```python
from build123d import *

# Parameters (mm, degrees)
F0_W     = 114.3
F0_H     = 152.4
F1_DEPTH = 15.24
F2_W     = 101.6
F2_H     = 14.1132464528
F3_DEPTH = 57.15
F4_DEPTH = 57.15
F6_DEPTH = 50.8
F7_DEPTH = 100.838


with BuildPart() as f1:
    # F0 (on Right) → F1 (new body)
    with BuildSketch(Plane.YZ):
        Rectangle(F0_W, F0_H)
    extrude(amount=F1_DEPTH)

    # F2 (on Front) → F3 (join)
    with BuildSketch(Plane.XZ):
        with Locations((66.04, -69.1433767736)):
            Rectangle(F2_W, F2_H)
    extrude(amount=F3_DEPTH)

    # F2 (on Front) → F4 (join)
    with BuildSketch(Plane.XZ):
        with Locations((66.04, -69.1433767736)):
            Rectangle(F2_W, F2_H)
    extrude(amount=-F4_DEPTH)

    # F5 (on Front) → F6 (join)
    with BuildSketch(Plane.XZ):
        with BuildLine():
            ThreePointArc((100.9056121111, 15.8293191344), (108.7441404523, 44.1781850532), (100.9056121111, 72.527050972))
            ThreePointArc((100.9056121111, 72.527050972), (58.597203119, 86.5942412093), (15.24, 76.2))
            Line((15.24, 76.2), (15.24, -62.0867535472))
            Line((15.24, -62.0867535472), (103.4958660603, -62.0867535472))
            ThreePointArc((103.4958660603, -62.0867535472), (119.3690519034, -22.5579711646), (100.9056121111, 15.8293191344))
        make_face()
        with BuildLine():
            Line((27.7020576755, -54.1285201907), (27.7020576755, 9.2299426906))
            Line((27.7020576755, 9.2299426906), (98.4420868913, 8.9223771356))
            ThreePointArc((98.4420868913, 8.9223771356), (110.4971458699, -23.121521712), (95.9815699021, -54.1285201907))
            Line((95.9815699021, -54.1285201907), (27.7020576755, -54.1285201907))
        make_face(mode=Mode.SUBTRACT)
        with BuildLine():
            ThreePointArc((95.6577137113, 66.4370954037), (102.0499654522, 45.5430957208), (98.4420868913, 23.9930767566))
            Line((98.4420868913, 23.9930767566), (25.8403848857, 23.9930767566))
            Line((25.8403848857, 23.9930767566), (25.8403848857, 72.8959664702))
            ThreePointArc((25.8403848857, 72.8959664702), (61.5459883334, 78.2810634281), (95.6577137113, 66.4370954037))
        make_face(mode=Mode.SUBTRACT)
    extrude(amount=F6_DEPTH)

    # F7 (add): a face of the model
    f7_faces = [f1.faces().sort_by_distance(p)[0] for p in [
        (106.9281796112, -50.8, 44.1781850532),
    ]]
    extrude(f7_faces, amount=-F7_DEPTH)


solid = f1.part
```
Verification items for the finished model (mm, model axes). A direction names the side the tool comes from. Coordinates: 2 decimals unless noted, no trailing zeros. Loops run counter-clockwise (first coordinate to the right, second up) from the corner with the lowest first, then second, coordinate; pieces in that order, holes last. Notation, with made-up numbers: (-8.5, 57) -> (41.5, 57) arc R22 ccw to (41.5, 74) -> close; hole circle Ø10 at (72.25, -10.5). An arc over 180 degrees is marked (long way). Answer in a Markdown table with one row per item. Add a question column.
1. Section check A-A, the plane z = 3. Enter the section's corners in (x, y), then the cut area to 3 significant figures.
2. Draft check along X on faces 4 (the face through (62, -1, -54.129)), 5 (the face through (59.229, -1.087, 86.565)), 6 (the face through (58, -1, -76.2)). Enter one of: +X half, -X half, draft (parallel to the pull), parting line (faces both ways), or undercut.
3. Depth check by flat-ended pin: P1, Ø3.5, axis at y = 55, z = -11, coming from the +X side; P2, Ø12, axis at y = 31.5, z = 35, coming from the +X side; P3, Ø17, axis at x = 7, y = 16, coming from the +Z side. Enter the tip coordinate at first touch or a pass-through.
4. Section check B-B, the plane x = 73. Enter the section's corners in (y, z).
5. Section check D-D, the plane z = -58. Enter the section's corners in (x, y).
6. Access from +Z, -Z, +X, -X, +Y, -Y to the whole of each face (thin tool, end or side, straight path). Record for faces 1 (the face through (59, 50.038, 13)), 2 (the face through (15.24, -54, 8)), 3 (the face through (63, -1, 23.993)).
7. Material ranges on probe 1 along Z at (x, y) = (60, -19); probe 2 along Z at (x, y) = (57, -36); probe 3 along X at (y, z) = (-15, -65), recorded low to high. Write a range as [from, to].
8. Section check C-C, the plane y = 44.5. Enter the section's corners in (x, z), then the cut area to 3 significant figures.
Derived:
| question | item | result |
|---|---|---|
| 1 | outline | (0, -57.15) -> (15.24, -57.15) -> (15.24, -50.8) -> (27.7, -50.8) -> (27.7, 50.04) -> (15.24, 50.04) -> (15.24, 57.15) -> (0, 57.15) -> close; (103.16, -50.8) -> (111.79, -50.8) -> (111.79, 50.04) -> (103.16, 50.04) -> close |
| 1 | area | 3,870 mm² |
| 2 | face 4 | undercut |
| 2 | face 5 | parting line |
| 2 | face 6 | draft |
| 3 | P1 | stops at x = 15.24 |
| 3 | P2 | stops at x = 108.65 |
| 3 | P3 | stops at z = 76.35 |
| 4 | outline | (-57.15, -76.2) -> (57.15, -76.2) -> (57.15, -62.09) -> (50.04, -62.09) -> (50.04, -54.13) -> (-50.8, -54.13) -> (-50.8, -62.09) -> (-57.15, -62.09) -> close; (-50.8, 9.03) -> (50.04, 9.03) -> (50.04, 23.99) -> (-50.8, 23.99) -> close; (-50.8, 76.32) -> (50.04, 76.32) -> (50.04, 84.68) -> (-50.8, 84.68) -> close |
| 5 | outline | (0, -57.15) -> (15.24, -57.15) -> (15.24, -50.8) -> (107.26, -50.8) -> (107.26, 50.04) -> (15.24, 50.04) -> (15.24, 57.15) -> (0, 57.15) -> close |
| 6 | face 1 | +Z, +X, +Y |
| 6 | face 2 | +Z, +X, -Y |
| 6 | face 3 | +Y, -Y |
| 7 | probe 1 | z = [-76.2, -54.13], [9.09, 23.99], [78.41, 86.52] |
| 7 | probe 2 | z = [-76.2, -54.13], [9.1, 23.99], [78.56, 86.65] |
| 7 | probe 3 | x = [0, 116.84] |
| 8 | outline | (0, -76.2) -> (116.84, -76.2) -> (116.84, -62.09) -> (103.5, -62.09) arc R52.81 ccw to (100.91, 15.83) arc R55.18 ccw to (100.91, 72.53) arc R81.19 ccw to (15.24, 76.2) -> (0, 76.2) -> close; hole (25.84, 23.99) -> (98.44, 23.99) arc R47.64 ccw to (95.66, 66.44) arc R75.36 ccw to (25.84, 72.9) -> close; hole (27.7, -54.13) -> (95.98, -54.13) arc R44.08 ccw to (98.44, 8.92) -> (27.7, 9.23) -> close |
| 8 | area | 8,710 mm² |
